from build123d import *

# Parameters (mm, degrees)
EXTRUDE1_DEPTH = 10
SKETCH7_R      = 1.5
EXTRUDE3_DEPTH = 6.625
SKETCH6_R      = 2.38125
SKETCH6_R_2    = 2.6
SKETCH6_R_3    = 6.35
SKETCH6_R_4    = 6
EXTRUDE2_DEPTH = 5
EXTRUDE4_DEPTH = 9
EXTRUDE5_DEPTH = 9


with BuildPart() as part:
    # Sketch5 → Extrude1 (new body)
    with BuildSketch(Plane.XY):
        with BuildLine():
            Line((-46.55, -2.6), (-46.55, -9.663597854))
            Line((-46.55, -9.663597854), (-39.925, -9.663597854))
            Line((-39.925, -9.663597854), (-39.925, 9.525))
            Line((-39.925, 9.525), (-46.55, 9.525))
            Line((-46.55, 9.525), (-46.55, 2.6))
            ThreePointArc((-46.55, 2.6), (-43.95, 0), (-46.55, -2.6))
        make_face()
    extrude(amount=EXTRUDE1_DEPTH)

    # Sketch7 → Extrude3 (cut)
    with BuildSketch(Plane(origin=(-39.925, 0, 0), x_dir=(0, 0, -1), z_dir=(1, 0, 0))):
        with Locations((-4.7625, 6.35)):
            Circle(SKETCH7_R)
        with Locations((-4.7625, -6.35)):
            Circle(SKETCH7_R)
    extrude(amount=-EXTRUDE3_DEPTH, mode=Mode.SUBTRACT)

    # Sketch6 → Extrude2 (add)
    with BuildSketch(Plane(origin=(0, 0, 0), x_dir=(-1, 0, 0), z_dir=(0, 0, -1))):
        Polygon((84.65, 38.1), (8.45, 38.1), (8.45, -38.1), (84.65, -37.995357572), align=None)
        with Locations((78.93, -32.38)):
            Circle(SKETCH6_R, mode=Mode.SUBTRACT)
        with Locations((14.17, -32.38)):
            Circle(SKETCH6_R, mode=Mode.SUBTRACT)
        with Locations((14.17, 32.38)):
            Circle(SKETCH6_R, mode=Mode.SUBTRACT)
        with Locations((78.93, 32.38)):
            Circle(SKETCH6_R, mode=Mode.SUBTRACT)
        with Locations((46.55, 0)):
            Circle(SKETCH6_R_2, mode=Mode.SUBTRACT)
        with Locations((69.85, -25.4)):
            Circle(SKETCH6_R_3, mode=Mode.SUBTRACT)
        with Locations((66.675, 25.4)):
            Circle(SKETCH6_R_3, mode=Mode.SUBTRACT)
        with Locations((25.4, 25.4)):
            Circle(SKETCH6_R_3, mode=Mode.SUBTRACT)
        with Locations((25.4, -25.4)):
            Circle(SKETCH6_R_3, mode=Mode.SUBTRACT)
        with Locations((58.7375, -6.35)):
            Circle(SKETCH6_R_4, mode=Mode.SUBTRACT)
        with Locations((58.7375, 6.35)):
            Circle(SKETCH6_R_4, mode=Mode.SUBTRACT)
        with Locations((31.75, -6.35)):
            Circle(SKETCH6_R_4, mode=Mode.SUBTRACT)
        with Locations((31.75, 6.35)):
            Circle(SKETCH6_R_4, mode=Mode.SUBTRACT)
    extrude(amount=EXTRUDE2_DEPTH)

    # Sketch9 → Extrude4 (add)
    with BuildSketch(Plane.XY):
        with BuildLine():
            Line((-53.175, -9.663597854), (-39.925, -9.663597854))
            ThreePointArc((-39.925, -9.663597854), (-46.55, -16.288597854), (-53.175, -9.663597854))
        make_face()
        with BuildLine():
            Line((-39.925, 9.525), (-53.175, 9.525))
            ThreePointArc((-53.175, 9.525), (-46.55, 16.15), (-39.925, 9.525))
        make_face()
    extrude(amount=EXTRUDE4_DEPTH)

    # Sketch10 → Extrude5 (cut)
    with BuildSketch(Plane.XY.offset(9)):
        Polygon((-46.55, 9.525), (-46.55, 9.725), (-53.997578108, 9.725), (-53.997578108, -9.863597854), (-46.55, -9.863597854), (-46.55, -9.663597854), align=None)
    extrude(amount=-EXTRUDE5_DEPTH, mode=Mode.SUBTRACT)


solid = part.part
Design review of the part built by this model. Coordinates are the model's own, in mm. A direction names the side the tool comes from. Coordinates: 2 decimals unless noted, no trailing zeros. Order: outer loops, then holes, each group sorted by start corner. A loop starts at its lowest first (then second) coordinate and runs counter-clockwise, first axis right, second up. Notation, with made-up numbers: M 84.25,5 L 100.25,5 A22 ccw 100.25,38 Z; hole C 10.25,-37.5 d4. An arc over 180 degrees is marked long. Use a Markdown table: item, result.
(1) For faces 1 (the cylindrical face through (-76.55, -32.28, -2.46)), 2 (the flat face through (-50, 9.725, 5)), list the 3-axis set-ups (+Z, -Z, +X, -X, +Y, -Y) from which the entire face can be reached by the end or side of a thin tool; tool diameter is ignored.
Worked answers:
| item | result |
|---|---|
| face 1 | +Z, -Z |
| face 2 | +Z, -X |
(2) For P1, Ø4, axis at y = -6.35, z = 4.76, coming from the +X side (3 decimals); P2, Ø10, axis at x = -47, y = -18.5, coming from the +Z side; P3, Ø3.5, axis at y = -5, z = 3.5, coming from the -X side, all flat-tipped, find the tip position at first contact; note any pin that passes through.
Worked answers:
| item | result |
|---|---|
| P1 | stops at x = -39.925 |
| P2 | stops at z = 9 |
| P3 | stops at x = -46.55 |
(3) Add section C-C (x = -36). Give the boundary of the cut face in (y, z).
Worked answers:
| item | result |
|---|---|
| outline | M -38.06,-5 L -10.59,-5 L -10.59,0 L -38.06,0 Z; M -2.11,-5 L 2.11,-5 L 2.11,0 L -2.11,0 Z; M 10.59,-5 L 38.1,-5 L 38.1,0 L 10.59,0 Z |
(4) Add section D-D (y = 13.5). Give the boundary of the cut face in (x, z), then the cut area to 3 significant figures.
Worked answers:
| item | result |
|---|---|
| outline | M -84.65,-5 L -8.45,-5 L -8.45,0 L -41.25,0 L -41.25,9 L -51.85,9 L -51.85,0 L -84.65,0 Z |
| area | 476 mm2 |
(5) Add section B-B (y = -25.4). Give the boundary of the cut face in (x, z).
Worked answers:
| item | result |
|---|---|
| outline | M -84.65,-5 L -76.2,-5 L -76.2,0 L -84.65,0 Z; M -63.5,-5 L -31.75,-5 L -31.75,0 L -63.5,0 Z; M -19.05,-5 L -8.45,-5 L -8.45,0 L -19.05,0 Z |
(6) Add section A-A (z = -4). Count the separate pieces of the cut face and the enclosed holes in it, then the cut area to 3 significant figures.
Worked answers:
| item | result |
|---|---|
| separate pieces | 1 |
| enclosed holes | 13 |
| area | 4,750 mm2 |
(7) Draft analysis for pull direction Y (two halves, no side actions). For faces 3 (the cylindrical face through (-46.306, -16.284, 4.437)), 4 (the cylindrical face through (-43.19, -5.34, 5.87)), 5 (the cylindrical face through (-72.54, 22.97, -2.46)), 6 (the flat face through (-46, -12, 9)), state which applies: released by +Y, released by -Y, zero draft, split by the parting line, or undercut.
Worked answers:
| item | result |
|---|---|
| face 3 | released by -Y |
| face 4 | undercut |
| face 5 | undercut |
| face 6 | zero draft |
(8) Wall thickness on probe 1 along Y at (x, z) = (-28.5, -3.5); probe 2 along Y at (x, z) = (-32.5, -3.75); probe 3 along Y at (x, z) = (-37, -1.75): over which ranges is each line inside the solid? List them lowest first.
Worked answers:
| item | result |
|---|---|
| probe 1 | y = -38.07 to -30.94, -19.86 to -11.39, -1.31 to 1.31, 11.39 to 19.86, 30.94 to 38.1 |
| probe 2 | y = -38.07 to -12.3, -0.4 to 0.4, 12.3 to 38.1 |
| probe 3 | y = -38.06 to -9.25, -3.45 to 3.45, 9.25 to 38.1 |
